Geometry check sheet. Reference: the model listing, model coordinates, mm. Face numbers are marked on the shaded views. A direction names the side the tool comes from. Coordinates: 2 decimals unless noted, no trailing zeros. Loops run counter-clockwise (first coordinate to the right, second up) from the corner with the lowest first, then second, coordinate; pieces in that order, holes last. Notation, with made-up numbers: M -24.75,65 L -16.75,65 A18 cw -16.75,69 Z; hole C 15,59 d4. An arc over 180 degrees is marked long. One line per question, with ' | ' between items. Start each with the question number.
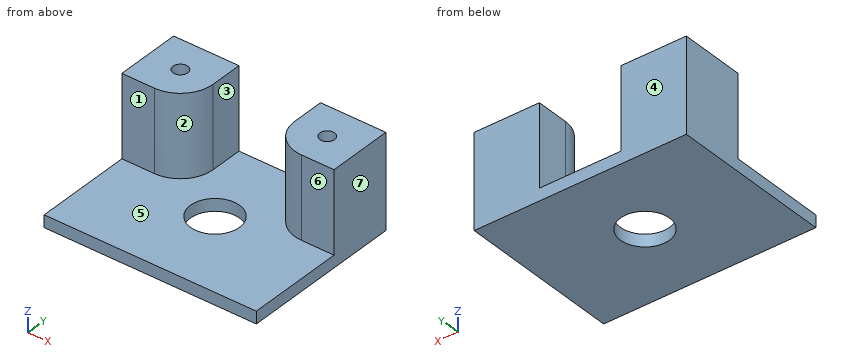
from build123d import *

# Parameters (mm, degrees)
F0_W     = 165.1
F0_H     = 127
F0_R     = 19.05
F1_DEPTH = 9.525
F3_DEPTH = 63.5
F5_D     = 11.50874
F5_DEPTH = 16.51
F5_TIP   = 3.4575743203


with BuildPart() as f1:
    # F0 (on Top) → F1 (new body)
    with BuildSketch(Plane.XY):
        Rectangle(F0_W, F0_H)
        Circle(F0_R, mode=Mode.SUBTRACT)
    extrude(amount=-F1_DEPTH)

    # F2 (on face) → F3 (join)
    with BuildSketch(Plane.XY):
        with BuildLine():
            Line((-31.75, 63.5), (-82.55, 63.5))
            Line((-82.55, 63.5), (-82.55, 12.7))
            Line((-82.55, 12.7), (-57.15, 12.7))
            ThreePointArc((-57.15, 12.7), (-39.1894877579, 20.1394877579), (-31.75, 38.1))
            Line((-31.75, 38.1), (-31.75, 63.5))
        make_face()
        with BuildLine():
            Line((82.55, 63.5), (31.75, 63.5))
            Line((31.75, 63.5), (31.75, 38.1))
            ThreePointArc((31.75, 38.1), (39.1894877579, 20.1394877579), (57.15, 12.7))
            Line((57.15, 12.7), (82.55, 12.7))
            Line((82.55, 12.7), (82.55, 63.5))
        make_face()
    extrude(amount=F3_DEPTH)

    # F5
    with Locations(Plane.XY.offset(63.5)):
        with Locations((57.15, 38.1), (-57.15, 38.1)):
            Hole(F5_D / 2, depth=F5_DEPTH)
            with Locations((0, 0, -(F5_DEPTH + F5_TIP / 2))):  # 118° drill point
                Cone(0, F5_D / 2, F5_TIP, mode=Mode.SUBTRACT)


solid = f1.part
1. Sectioned sample at D-D (z = 35). Record the cut outline in (x, y), and give its area (3 significant figures).
2. Sectioned sample at B-B (y = 0). Record the cut outline in (x, z) (3 decimals), and give its area (3 significant figures).
3. Sectioned sample at C-C (x = 0). Record the cut outline in (y, z) (3 decimals), and give its area (3 significant figures).
4. Depth check by flat-ended pin: pin 1 Ø20.5 at (x, z) = (-76, 18) entering from -Y; pin 2 Ø10.5 at (x, y) = (-57.15, 38.1) entering from +Z. Enter the tip coordinate at first touch or a pass-through.
5. Sectioned sample at A-A (z = 52). Record the cut outline in (x, y).
6. Tool access check on the marked faces 1, 2, 3 and 4. Record the directions out of +Z, -Z, +X, -X, +Y, -Y that give a thin tool (end or side, any length) a straight path to the whole face; none if there is none.
7. Draft check along X on the marked faces 5, 6 and 7. Enter one of: +X half, -X half, draft (parallel to the pull), parting line (faces both ways), or undercut.
8. Thickness scan on line 1 (X direction, y = 38.1, z = 60); line 2 (Y direction, x = -57, z = 56); line 3 (Y direction, x = 0, z = -3.75). Record the ranges inside material, lowest first.
Result:
1) outline: M -82.55,12.7 L -57.15,12.7 A25.4 ccw -31.75,38.1 L -31.75,63.5 L -82.55,63.5 Z; M 31.75,38.1 A25.4 ccw 57.15,12.7 L 82.55,12.7 L 82.55,63.5 L 31.75,63.5 Z | area: 4,880 mm2
2) outline: M -82.55,-9.525 L -19.05,-9.525 L -19.05,0 L -82.55,0 Z; M 19.05,-9.525 L 82.55,-9.525 L 82.55,0 L 19.05,0 Z | area: 1,210 mm2
3) outline: M -63.5,-9.525 L -19.05,-9.525 L -19.05,0 L -63.5,0 Z; M 19.05,-9.525 L 63.5,-9.525 L 63.5,0 L 19.05,0 Z | area: 847 mm2
4) pin 1: stops at y = 12.7 | pin 2: stops at z = 46.69
5) outline: M -82.55,12.7 L -57.15,12.7 A25.4 ccw -31.75,38.1 L -31.75,63.5 L -82.55,63.5 Z; M 31.75,38.1 A25.4 ccw 57.15,12.7 L 82.55,12.7 L 82.55,63.5 L 31.75,63.5 Z; hole C -57.15,38.1 d11.51; hole C 57.15,38.1 d11.51
6) face 1: +Z, +X, -X, -Y | face 2: +Z, -Y | face 3: +Z, +Y, -Y | face 4: +Z, -Z, +X, -X, +Y
7) face 5: undercut | face 6: draft | face 7: +X half
8) line 1: x = -82.55 to -62.9, -51.4 to -31.75, 31.75 to 51.4, 62.9 to 82.55 | line 2: y = 12.7 to 32.35, 43.85 to 63.5 | line 3: y = -63.5 to -19.05, 19.05 to 63.5
